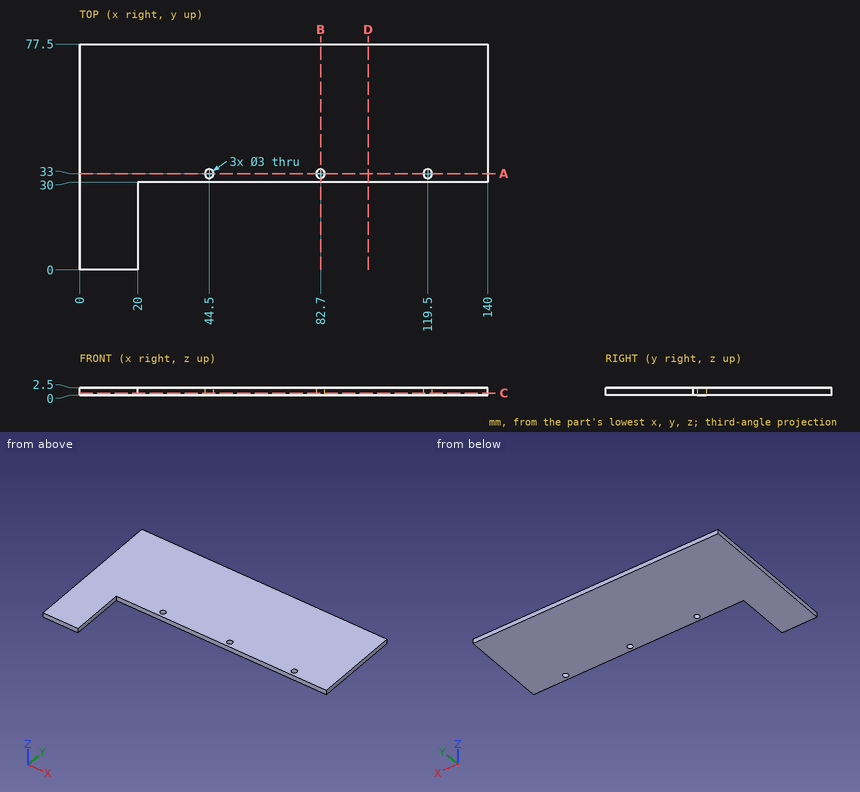
Source: three-view drawing plus pictorial views. Frame: mm from the lowest corner of the part. Coordinates: 2 decimals unless noted, no trailing zeros. Order: outer loops, then holes, each group sorted by start corner. A loop starts at its lowest first (then second) coordinate and runs counter-clockwise, first axis right, second up.
Item 1: First-contact query: P1, Ø0.8, axis at y = 10, z = 1, coming from the +X side. Flat tip, straight axial feed; report the tip coordinate or a pass-through.
Output values:
P1: stops at x = 20
Item 2: Cut plane B-B (x = 82.7). Return loops of the section in (y, z), plus the area to 3 significant figures.
Output values:
outline: (30, 0) - (31.5, 0) - (31.5, 2.5) - (30, 2.5) - close; (34.5, 0) - (77.5, 0) - (77.5, 2.5) - (34.5, 2.5) - close
area: 111 mm2
Item 3: Cut plane A-A (y = 33). Return loops of the section in (x, z).
Output values:
outline: (0, 0) - (43, 0) - (43, 2.5) - (0, 2.5) - close; (46, 0) - (81.2, 0) - (81.2, 2.5) - (46, 2.5) - close; (84.2, 0) - (118, 0) - (118, 2.5) - (84.2, 2.5) - close; (121, 0) - (140, 0) - (140, 2.5) - (121, 2.5) - close
Item 4: Cut plane C-C (z = 0.75). Return loops of the section in (x, y).
Output values:
outline: (0, 0) - (20, 0) - (20, 30) - (140, 30) - (140, 77.5) - (0, 77.5) - close; hole circle Ø3 at (44.5, 33); hole circle Ø3 at (82.7, 33); hole circle Ø3 at (119.5, 33)
Item 5: Cut plane D-D (x = 99). Return loops of the section in (y, z), plus the area to 3 significant figures.
Output values:
outline: (30, 0) - (77.5, 0) - (77.5, 2.5) - (30, 2.5) - close
area: 119 mm2
Item 6: Material intervals for line 1 (Y direction, x = 119.5, z = 1.65); line 2 (Y direction, x = 56.5, z = 0.9), sorted ascending.
Output values:
line 1: y = 30 to 31.5, 34.5 to 77.5
line 2: y = 30 to 77.5
